Read the model definition and answer for the solid it produces. Units are mm, in the model's axes. Coordinates: 2 decimals unless noted, no trailing zeros. Order: outer loops, then holes, each group sorted by start corner. A loop starts at its lowest first (then second) coordinate and runs counter-clockwise, first axis right, second up.
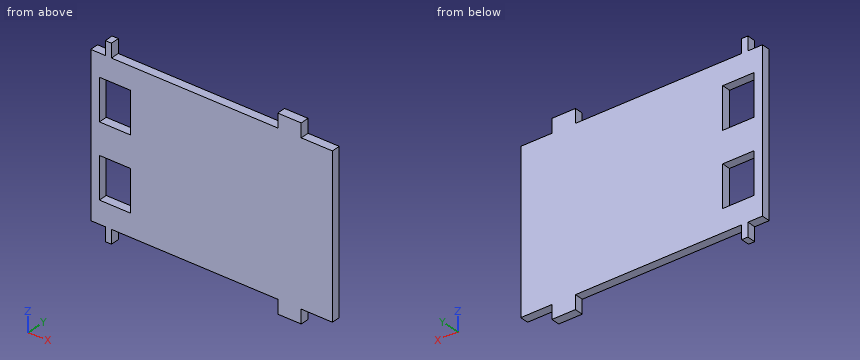
```python
from build123d import *

# Parameters (mm, degrees)
SKETCH_1_W          = 70
SKETCH_1_H          = 54
EXTRUDE_1_DEPTH     = 2.5
SKETCH_2_W          = 9.03
SKETCH_2_H          = 4
SKETCH_2_W_2        = 48.17
SKETCH_2_W_3        = 4.2
CUT_EXTRUDE_1_DEPTH = 3.5
SKETCH_3_W          = 9
SKETCH_3_H          = 12
CUT_EXTRUDE_2_DEPTH = 3.5


with BuildPart() as part:
    # 草图1 → 凸台-拉伸1 (new body)
    with BuildSketch(Plane(origin=(0, 0, 0), x_dir=(1, 0, 0), z_dir=(0, 1, 0))):
        Rectangle(SKETCH_1_W, SKETCH_1_H)
    extrude(amount=EXTRUDE_1_DEPTH)

    # 草图2 → 切除-拉伸1 (cut, through all)
    with BuildSketch(Plane(origin=(0, 2.5, 0), x_dir=(1, 0, 0), z_dir=(0, 1, 0))):
        with Locations((30.485, 25)):
            Rectangle(SKETCH_2_W, SKETCH_2_H)
        with Locations((-4.915, 25)):
            Rectangle(SKETCH_2_W_2, SKETCH_2_H)
        with Locations((-32.9, 25)):
            Rectangle(SKETCH_2_W_3, SKETCH_2_H)
        with Locations((-32.9, -25)):
            Rectangle(SKETCH_2_W_3, SKETCH_2_H)
        with Locations((30.485, -25)):
            Rectangle(SKETCH_2_W, SKETCH_2_H)
        with Locations((-4.915, -25)):
            Rectangle(SKETCH_2_W_2, SKETCH_2_H)
    extrude(amount=-CUT_EXTRUDE_1_DEPTH, mode=Mode.SUBTRACT)

    # 草图3 → 切除-拉伸2 (cut, through all)
    with BuildSketch(Plane(origin=(0, 2.5, 0), x_dir=(1, 0, 0), z_dir=(0, 1, 0))):
        with Locations((-28, 10.5)):
            Rectangle(SKETCH_3_W, SKETCH_3_H)
        with Locations((-28, -10.5)):
            Rectangle(SKETCH_3_W, SKETCH_3_H)
    extrude(amount=-CUT_EXTRUDE_2_DEPTH, mode=Mode.SUBTRACT)


solid = part.part
```
1) A cutting plane is placed at B-B, the plane y = 0.9. Determine the outline of the cut face in (x, z).
A:
outline: (-35, -23) - (-30.8, -23) - (-30.8, -27) - (-29, -27) - (-29, -23) - (19.17, -23) - (19.17, -27) - (25.97, -27) - (25.97, -23) - (35, -23) - (35, 23) - (25.97, 23) - (25.97, 27) - (19.17, 27) - (19.17, 23) - (-29, 23) - (-29, 27) - (-30.8, 27) - (-30.8, 23) - (-35, 23) - close; hole (-32.5, -16.5) - (-23.5, -16.5) - (-23.5, -4.5) - (-32.5, -4.5) - close; hole (-32.5, 4.5) - (-23.5, 4.5) - (-23.5, 16.5) - (-32.5, 16.5) - close
2) A cutting plane is placed at A-A, the plane z = 11. Determine the outline of the cut face in (x, y).
A:
outline: (-35, 0) - (-32.5, 0) - (-32.5, 2.5) - (-35, 2.5) - close; (-23.5, 0) - (35, 0) - (35, 2.5) - (-23.5, 2.5) - close
3) Flat-ended cylindrical pins translate along their axes: pin 1 Ø1.2 at (x, y) = (32.5, 2) entering from -Z; pin 2 Ø0.8 at (y, z) = (1, 25.5) entering from -X; pin 3 Ø0.8 at (y, z) = (0.5, -26) entering from +X; pin 4 Ø3 at (x, z) = (-4.5, -21.5) entering from -Y. Find the tip coordinate at first contact, or state that the pin passes through.
A:
pin 1: stops at z = -23
pin 2: stops at x = -30.8
pin 3: stops at x = 25.97
pin 4: stops at y = 0
4) A cutting plane is placed at C-C, the plane x = -13. Determine the outline of the cut face in (y, z).
A:
outline: (0, -23) - (2.5, -23) - (2.5, 23) - (0, 23) - close
5) Straight lines are drawn through the part: line 1 (X direction, y = 1.7, z = 13.5); line 2 (Z direction, x = -25.5, y = 2.1); line 3 (Z direction, x = -29.5, y = 0.8). For each, find the intervals that lie inside material, in ascending order.
A:
line 1: x = -35 to -32.5, -23.5 to 35
line 2: z = -23 to -16.5, -4.5 to 4.5, 16.5 to 23
line 3: z = -27 to -16.5, -4.5 to 4.5, 16.5 to 27
